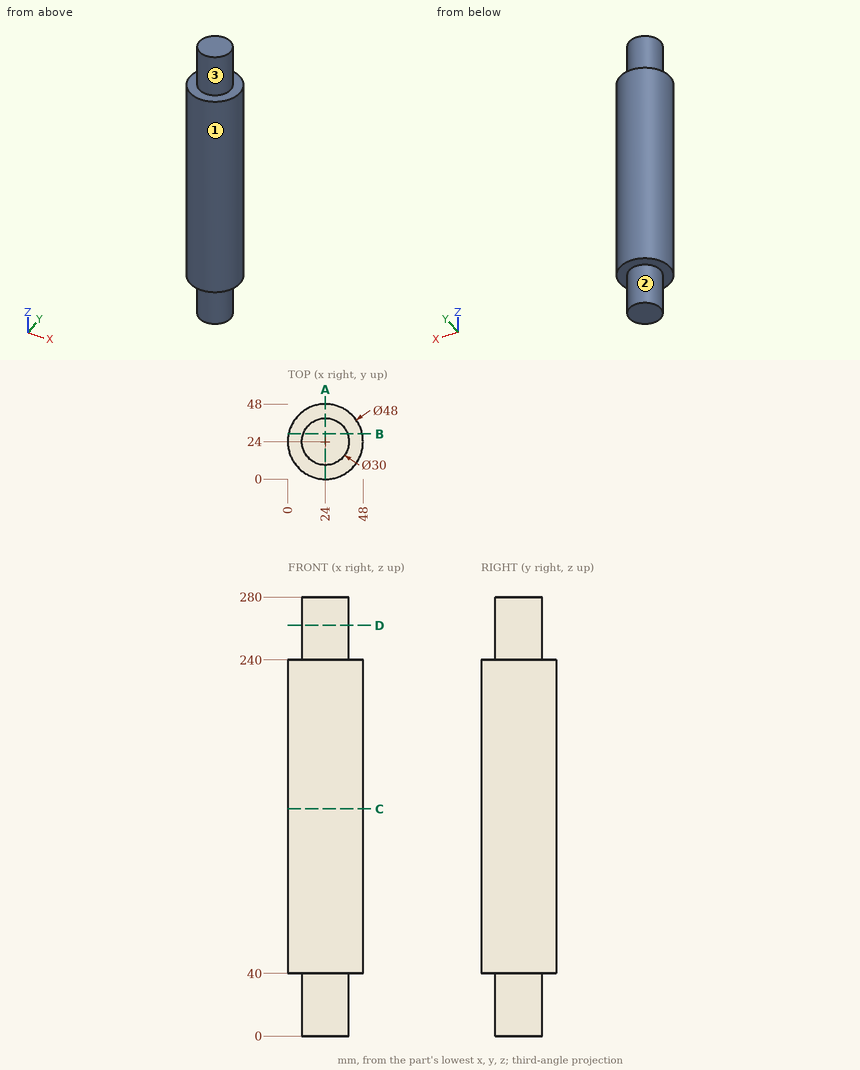
Design review of the part shown in the three views and the two pictorial views. Dimensions are in mm from the part's minimum x, y and z. A direction names the side the tool comes from. Give positions to 0.01 mm unless a question says otherwise; leave off trailing zeros. Write each loop counter-clockwise with the first axis right and the second up, starting at its lowest first coordinate (ties: lowest second). Pieces come first, ordered by that corner, then holes. Notation, with made-up numbers: M -4.75,80.5 L 11.25,80.5 A12 cw 11.25,100.5 Z; hole C 62.5,23.5 d5. An arc over 180 degrees is marked long. Answer as CSV lines item,"result".
1. For pin 1 (1 mm diameter, centred on x = 23, y = 6, fed in from -Z); pin 2 (5 mm diameter, centred on x = 9.5, z = 164, fed in from +Y); pin 3 (1.5 mm diameter, centred on x = 28.5, z = 224, fed in from -Y), all flat-tipped, find the tip position at first contact; note any pin that passes through.
Findings:
pin 1,"stops at z = 40"
pin 2,"stops at y = 44.78"
pin 3,"stops at y = 0.29"
2. Consider section B-B, the plane y = 29. Write out the cut boundary in (x, z).
Findings:
outline,"M 0.53,40 L 9.86,40 L 9.86,0 L 38.14,0 L 38.14,40 L 47.47,40 L 47.47,240 L 38.14,240 L 38.14,280 L 9.86,280 L 9.86,240 L 0.53,240 Z"
3. Wall thickness on line 1 (Z direction, x = 14, y = 44.5); line 2 (Y direction, x = 30, z = 24.5); line 3 (Y direction, x = 45, z = 174): over which ranges is each line inside the solid? List them lowest first.
Findings:
line 1,"z = 40 to 240"
line 2,"y = 10.25 to 37.75"
line 3,"y = 12.38 to 35.62"
4. For the marked faces 1, 2 and 3, list the 3-axis set-ups (+Z, -Z, +X, -X, +Y, -Y) from which the entire face can be reached by the end or side of a thin tool; tool diameter is ignored.
Findings:
face 1,"+Z, -Z"
face 2,"-Z"
face 3,"+Z"
5. Consider section A-A, the plane x = 24. Write out the cut boundary in (y, z).
Findings:
outline,"M 0,40 L 9,40 L 9,0 L 39,0 L 39,40 L 48,40 L 48,240 L 39,240 L 39,280 L 9,280 L 9,240 L 0,240 Z"
6. Consider section C-C, the plane z = 145. Write out the cut boundary in (x, y).
Findings:
outline,"C 24,24 d48"
7. Consider section D-D, the plane z = 262. Write out the cut boundary in (x, y), then the cut area to 3 significant figures.
Findings:
outline,"C 24,24 d30"
area,"707 mm2"
